Design review of the part built by this model. Coordinates are the model's own, in mm. Face numbers are marked on the shaded views. A direction names the side the tool comes from. Coordinates: 2 decimals unless noted, no trailing zeros. Write each loop counter-clockwise with the first axis right and the second up, starting at its lowest first coordinate (ties: lowest second). Pieces come first, ordered by that corner, then holes. Notation, with made-up numbers: (38, -22.5) - (81, -22.5) arc R9 cw to (81, -15.5) - close; hole circle Ø2 at (59, -27). An arc over 180 degrees is marked (long way). Use a Markdown table: item, result.
from build123d import *

# Parameters (mm, degrees)
SKETCH_1_W          = 36
SKETCH_1_H          = 32
SKETCH_1_R          = 1.6
EXTRUDE_1_DEPTH     = 4
EXTRUDE_2_DEPTH     = 32
SKETCH_8_R          = 1.6
CUT_EXTRUDE_1_DEPTH = 53.619768148
SKETCH1_W           = 4
SKETCH1_H           = 32
BOSS_EXTRUDE1_DEPTH = 3
SKETCH2_W           = 5
SKETCH2_H           = 32
BOSS_EXTRUDE2_DEPTH = 12
CUT_EXTRUDE1_DEPTH  = 5
BOSS_EXTRUDE5_DEPTH = 5
BOSS_EXTRUDE6_START = 3
SKETCH7_W           = 15
SKETCH7_H           = 32
SKETCH7_R           = 1.6
BOSS_EXTRUDE6_DEPTH = 3
CUT_EXTRUDE2_DEPTH  = 0.25
BOSS_EXTRUDE7_START = 2.5
SKETCH9_W           = 15
SKETCH9_H           = 32
SKETCH9_R           = 1.6
BOSS_EXTRUDE7_DEPTH = 2.5
BOSS_EXTRUDE8_DEPTH = 2.5
CUT_EXTRUDE3_DEPTH  = 2.5
FILLET2_R           = 3
FILLET4_R           = 3
FILLET5_R           = 3
FILLET9_R           = 1
FILLET11_R          = 1
CUT_EXTRUDE4_DEPTH  = 3
CUT_EXTRUDE5_DEPTH  = 3
FILLET14_R          = 1


with BuildPart() as part:
    # Эскиз1 → Бобышка-Вытянуть1 (new body)
    with BuildSketch(Plane.XY):
        with Locations((18, 16)):
            Rectangle(SKETCH_1_W, SKETCH_1_H)
        with Locations((8, 26)):
            Circle(SKETCH_1_R, mode=Mode.SUBTRACT)
        with Locations((28, 26)):
            Circle(SKETCH_1_R, mode=Mode.SUBTRACT)
        with Locations((8, 6)):
            Circle(SKETCH_1_R, mode=Mode.SUBTRACT)
        with Locations((28, 6)):
            Circle(SKETCH_1_R, mode=Mode.SUBTRACT)
    extrude(amount=EXTRUDE_1_DEPTH)

    # Эскиз7 → Бобышка-Вытянуть2 (add)
    with BuildSketch(Plane(origin=(0, 32, 0), x_dir=(1, 0, 0), z_dir=(0, 1, 0))):
        Polygon((0, 0), (-1.2, 0), (-1.2, 15), (-5.2, 15), (-5.2, -19), (-1.2, -19), (-1.2, -4), (0, -4), align=None)
    extrude(amount=-EXTRUDE_2_DEPTH)

    # Эскиз8 → Вырез-Вытянуть1 (cut, through all)
    with BuildSketch(Plane(origin=(-1.2, 0, 0), x_dir=(0, 0, -1), z_dir=(1, 0, 0))):
        with Locations(Location((8, 24, 0), (0, 0, 90))):
            Circle(SKETCH_8_R)
        with Locations(Location((8, 8, 0), (0, 0, 90))):
            Circle(SKETCH_8_R)
        with Locations(Location((-12, 8, 0), (0, 0, 90))):
            Circle(SKETCH_8_R)
        with Locations(Location((-12, 24, 0), (0, 0, 90))):
            Circle(SKETCH_8_R)
    extrude(amount=-CUT_EXTRUDE_1_DEPTH, mode=Mode.SUBTRACT)

    # Sketch1 → Boss-Extrude1 (add)
    with BuildSketch(Plane(origin=(36, 0, 0), x_dir=(0, 0, -1), z_dir=(1, 0, 0))):
        with Locations((-2, 16)):
            Rectangle(SKETCH1_W, SKETCH1_H)
    extrude(amount=BOSS_EXTRUDE1_DEPTH)

    # Sketch2 → Boss-Extrude2 (add)
    with BuildSketch(Plane(origin=(0, 0, 0), x_dir=(-1, 0, 0), z_dir=(0, 0, -1))):
        with Locations((-36.5, 16)):
            Rectangle(SKETCH2_W, SKETCH2_H)
    extrude(amount=BOSS_EXTRUDE2_DEPTH)

    # Sketch3 → Cut-Extrude1 (cut)
    with BuildSketch(Plane(origin=(39, 0, 0), x_dir=(0, 0, -1), z_dir=(1, 0, 0))):
        Polygon((7, 32), (12, 32), (12, 23.339745962), align=None)
        Polygon((12, 8.660254038), (7, 0), (12, 0), align=None)
    extrude(amount=-CUT_EXTRUDE1_DEPTH, mode=Mode.SUBTRACT)

    # Sketch6 → Boss-Extrude5 (add)
    with BuildSketch(Plane(origin=(39, 0, 0), x_dir=(0, 0, -1), z_dir=(1, 0, 0))):
        Polygon((-16, 8.660254038), (-11, 0), (-4, 0), (-4, 32), (-11, 32), (-16, 23.339745962), align=None)
    extrude(amount=-BOSS_EXTRUDE5_DEPTH)

    # Sketch7 → Boss-Extrude6 (add)
    # profile 1 of 2: a face of its own
    with BuildSketch(Plane(origin=(-1.2, 0, 0), x_dir=(0, 0, -1), z_dir=(1, 0, 0)).offset(BOSS_EXTRUDE6_START)):
        with Locations((7.5, 16)):
            Rectangle(SKETCH7_W, SKETCH7_H)
        with Locations(Location((8, 24, 0), (0, 0, 90))):
            Circle(SKETCH7_R, mode=Mode.SUBTRACT)
        with Locations(Location((8, 8, 0), (0, 0, 90))):
            Circle(SKETCH7_R, mode=Mode.SUBTRACT)
    # profile 2 of 2: a face of its own
    with BuildSketch(Plane(origin=(-1.2, 0, 0), x_dir=(0, 0, -1), z_dir=(1, 0, 0)).offset(BOSS_EXTRUDE6_START)):
        with Locations((-11.5, 16)):
            Rectangle(SKETCH7_W, SKETCH7_H)
        with Locations(Location((-12, 24, 0), (0, 0, 90))):
            Circle(SKETCH7_R, mode=Mode.SUBTRACT)
        with Locations(Location((-12, 8, 0), (0, 0, 90))):
            Circle(SKETCH7_R, mode=Mode.SUBTRACT)
    extrude(amount=-BOSS_EXTRUDE6_DEPTH)

    # Sketch8 → Cut-Extrude2 (cut)
    with BuildSketch(Plane.ZY.offset(-34)):
        Polygon((-12, 23.339745962), (-12, 8.660254038), (-7, 0), (0, 0), (0, 32), (-7, 32), align=None)
        Polygon((4, 32), (4, 0), (11, 0), (16, 8.660254038), (16, 23.339745962), (11, 32), align=None)
    extrude(amount=-CUT_EXTRUDE2_DEPTH, mode=Mode.SUBTRACT)

    # Sketch9 → Boss-Extrude7 (add)
    with BuildSketch(Plane(origin=(1.8, 0, 0), x_dir=(0, 0, -1), z_dir=(1, 0, 0)).offset(BOSS_EXTRUDE7_START)):
        with Locations((7.5, 16)):
            Rectangle(SKETCH9_W, SKETCH9_H)
        with Locations(Location((8, 24, 0), (0, 0, 90))):
            Circle(SKETCH9_R, mode=Mode.SUBTRACT)
        with Locations(Location((8, 8, 0), (0, 0, 90))):
            Circle(SKETCH9_R, mode=Mode.SUBTRACT)
    extrude(amount=-BOSS_EXTRUDE7_DEPTH)

    # Sketch10 → Boss-Extrude8 (add)
    with BuildSketch(Plane.ZY.offset(-34.25)):
        Polygon((-7, 32), (-12, 23.339745962), (-12, 8.660254038), (-7, 0), (0, 0), (0, 32), align=None)
    extrude(amount=BOSS_EXTRUDE8_DEPTH)

    # Sketch11 → Cut-Extrude3 (cut)
    with BuildSketch(Plane.ZY.offset(-31.75)):
        Polygon((-7, 32), (-12, 23.339745962), (-12, 8.660254038), (-7, 0), align=None)
    extrude(amount=-CUT_EXTRUDE3_DEPTH, mode=Mode.SUBTRACT)

    # Fillet2
    # the kernel refuses this fillet: 3 mm, written as the material it takes off along each edge
    with BuildSketch(Plane(origin=(31.75, -7.395099729, -7), x_dir=(1, 0, 0), z_dir=(0, 1, 0))) as fillet2_piece_1:
        with BuildLine():
            CenterArc((3, -2.958039892), FILLET2_R, 99.594068227, 80.405931773)
            Line((0, -2.958039892), (-0.06, -2.958039892))
            Line((-0.06, -2.958039892), (-0.06, 0))
            Line((-0.06, 0), (0, 0.06))
            ThreePointArc((0, 0.06), (1.25, 0.06), (2.49, 0.059160798))
            Line((2.49, 0.059160798), (2.5, 0))
        make_face()
    extrude(amount=46.790199458, mode=Mode.SUBTRACT)

    # Fillet4
    fillet4_edges = [part.edges().sort_by_distance(p)[0] for p in [
        (36.625, 32, -7),
        (36.625, 0, -7),
        (36.625, 8.660254038, -12),
        (36.625, 23.339745962, -12),
    ]]
    fillet(fillet4_edges, radius=FILLET4_R)

    # Fillet5
    fillet5_edges = [part.edges().sort_by_distance(p)[0] for p in [
        (36.625, 32, 11),
        (36.625, 23.339745962, 16),
        (36.625, 8.660254038, 16),
        (36.625, 0, 11),
    ]]
    fillet(fillet5_edges, radius=FILLET5_R)

    # Fillet9
    fillet9_edges = [part.edges().sort_by_distance(p)[0] for p in [
        (39, 4.732050808, -9.732050808),
        (39, 16, -12),
        (39, 27.267949192, -9.732050808),
        (39, 32, 2),
        (39, 31.598076211, -6.767949192),
        (39, 23.31235552, -11.897777479),
        (39, 8.68764448, -11.897777479),
        (39, 0.401923789, -6.767949192),
        (39, 4.732050808, 13.732050808),
        (39, 0, 2),
        (39, 27.267949192, 13.732050808),
        (39, 16, 16),
        (39, 31.598076211, 10.767949192),
        (39, 23.31235552, 15.897777479),
        (39, 8.68764448, 15.897777479),
        (39, 0.401923789, 10.767949192),
    ]]
    fillet(fillet9_edges, radius=FILLET9_R)

    # Fillet11
    fillet11_edges = [part.edges().sort_by_distance(p)[0] for p in [
        (1.8, 16, 19),
        (-5.2, 16, 19),
        (-1.7, 32, 19),
        (-1.7, 0, 19),
    ]]
    fillet(fillet11_edges, radius=FILLET11_R)

    # Sketch12 → Cut-Extrude4 (cut)
    with BuildSketch(Plane(origin=(4.3, 0, 0), x_dir=(0, 0, -1), z_dir=(1, 0, 0))):
        Polygon((6.354551733, 26.85), (4.709103466, 24), (6.354551733, 21.15), (9.645448267, 21.15), (11.290896534, 24), (9.645448267, 26.85), align=None)
        Polygon((6.354551733, 10.85), (4.709103466, 8), (6.354551733, 5.15), (9.645448267, 5.15), (11.290896534, 8), (9.645448267, 10.85), align=None)
    extrude(amount=-CUT_EXTRUDE4_DEPTH, mode=Mode.SUBTRACT)

    # Sketch13 → Cut-Extrude5 (cut)
    with BuildSketch(Plane(origin=(1.8, 0, 0), x_dir=(0, 0, -1), z_dir=(1, 0, 0))):
        Polygon((-15.290896534, 24), (-13.645448267, 21.15), (-10.354551733, 21.15), (-8.709103466, 24), (-10.354551733, 26.85), (-13.645448267, 26.85), align=None)
        Polygon((-15.290896534, 8), (-13.645448267, 5.15), (-10.354551733, 5.15), (-8.709103466, 8), (-10.354551733, 10.85), (-13.645448267, 10.85), align=None)
    extrude(amount=-CUT_EXTRUDE5_DEPTH, mode=Mode.SUBTRACT)

    # Fillet14
    # the kernel refuses this fillet: 1 mm, written as the material it takes off along each edge
    with BuildSketch(Plane(origin=(-4.2, 1, 18), x_dir=(-1, 0, 0), z_dir=(0, -1, 0))) as fillet14_piece_1_section:
        Polygon((0, 0), (FILLET14_R, 0), (FILLET14_R, -FILLET14_R), (0, -FILLET14_R), align=None)
    fillet14_piece_1 = extrude(amount=FILLET14_R, mode=Mode.PRIVATE)
    fillet14_piece_1 = fillet14_piece_1 - Plane(origin=(-4.2, 1, 18), x_dir=(0.7071067811865475, 0, -0.7071067811865475), z_dir=(0, -1, 0)) * Sphere(FILLET14_R, mode=Mode.PRIVATE)
    add(fillet14_piece_1, mode=Mode.SUBTRACT)
    with BuildSketch(Plane(origin=(-4.2, 31, 18), x_dir=(0, 1, 0), z_dir=(-1, 0, 0))) as fillet14_piece_2_section:
        Polygon((0, 0), (FILLET14_R, 0), (FILLET14_R, -FILLET14_R), (0, -FILLET14_R), align=None)
    fillet14_piece_2 = extrude(amount=FILLET14_R, mode=Mode.PRIVATE)
    fillet14_piece_2 = fillet14_piece_2 - Plane(origin=(-4.2, 31, 18), x_dir=(0, -0.7071067811865475, -0.7071067811865475), z_dir=(-1, 0, 0)) * Sphere(FILLET14_R, mode=Mode.PRIVATE)
    add(fillet14_piece_2, mode=Mode.SUBTRACT)
    with BuildSketch(Plane(origin=(4.3, 32, -17.5), x_dir=(0, -1, 0), z_dir=(0, 0, 1))) as fillet14_piece_3:
        with BuildLine():
            CenterArc((FILLET14_R, -FILLET14_R), FILLET14_R, 90, 90)
            Line((0, -FILLET14_R), (0, 0))
            Line((0, 0), (FILLET14_R, 0))
        make_face()
    extrude(amount=17.5, mode=Mode.SUBTRACT)
    with BuildSketch(Plane(origin=(4.3, 0, 0), x_dir=(-1, 0, 0), z_dir=(0, 0, -1))) as fillet14_piece_4:
        with BuildLine():
            CenterArc((FILLET14_R, FILLET14_R), FILLET14_R, 180, 90)
            Line((0, FILLET14_R), (0, 0))
            Line((0, 0), (FILLET14_R, 0))
        make_face()
    extrude(amount=17.5, mode=Mode.SUBTRACT)
    with BuildSketch(Plane(origin=(4.3, -2.5, -15), x_dir=(-1, 0, 0), z_dir=(0, 1, 0))) as fillet14_piece_5:
        with BuildLine():
            CenterArc((FILLET14_R, FILLET14_R), FILLET14_R, 180, 90)
            Line((0, FILLET14_R), (0, 0))
            Line((0, 0), (FILLET14_R, 0))
        make_face()
    extrude(amount=37, mode=Mode.SUBTRACT)
    with BuildSketch(Plane(origin=(-5.2, 34.5, -15), x_dir=(0, 0, 1), z_dir=(0, -1, 0))) as fillet14_piece_6:
        with BuildLine():
            CenterArc((FILLET14_R, -FILLET14_R), FILLET14_R, 90, 90)
            Line((0, -FILLET14_R), (0, 0))
            Line((0, 0), (FILLET14_R, 0))
        make_face()
    extrude(amount=37, mode=Mode.SUBTRACT)
    with BuildSketch(Plane(origin=(-5.2, 32, -17.5), x_dir=(0, -1, 0), z_dir=(0, 0, 1)), Plane(origin=(-5.2, 0, -17.5), x_dir=(1, 0, 0), z_dir=(0, 0, 1))) as fillet14_piece_7:
        with BuildLine():
            CenterArc((FILLET14_R, FILLET14_R), FILLET14_R, 180, 90)
            Line((0, FILLET14_R), (0, 0))
            Line((0, 0), (FILLET14_R, 0))
        make_face()
    extrude(amount=35.5, mode=Mode.SUBTRACT)


solid = part.part
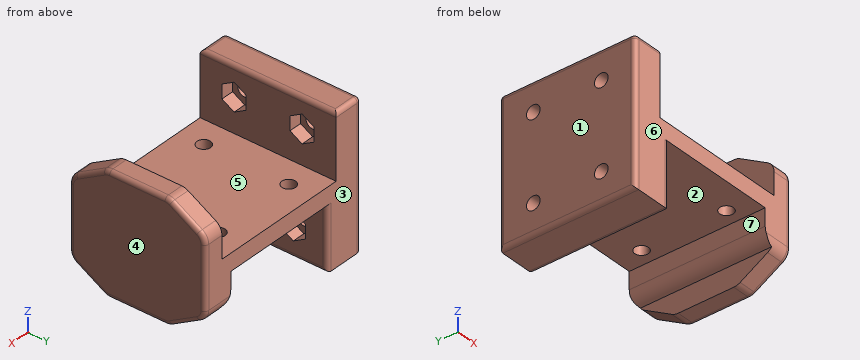
(1) Machinability: for the marked faces 5, 6 and 7, which of the approach directions +Z, -Z, +X, -X, +Y, -Y give a long, thin tool a straight path to every point of the face, cutting with its end or side? Answer none if there is none.
Determined:
| item | result |
|---|---|
| face 5 | +Z, +Y, -Y |
| face 6 | +Z, -Z, +X, -X, -Y |
| face 7 | -Z, +Y, -Y |
(2) For L1, parallel to Z at x = 0.25, y = 24; L2, parallel to Z at x = -3.3, y = 24; L3, parallel to X at y = 26.5, z = -3, list the stretches that pass through material, from the lowest coordinate up. Write a range as from..to.
Determined:
| item | result |
|---|---|
| L1 | -15..-9.6, -6.4..8.71, 15.29..19 |
| L2 | -15..-9.6, -6.4..10.4, 13.6..19 |
| L3 | -5.2..4.3, 31.75..39 |
(3) For pin 1 (5 mm diameter, centred on y = 24, z = -8, fed in from -X); pin 2 (6 mm diameter, centred on x = 9.5, y = 16.5, fed in from -Z); pin 3 (1.5 mm diameter, centred on x = 34, y = 25.5, fed in from -Z); pin 4 (1.1 mm diameter, centred on x = 36, y = 19, fed in from +Z), all flat-tipped, find the tip position at first contact; note any pin that passes through.
Determined:
| item | result |
|---|---|
| pin 1 | x = -5.2 |
| pin 2 | z = 0 |
| pin 3 | z = -11.16 |
| pin 4 | z = 16 |
(4) Draft analysis for pull direction X (two halves, no side actions). For the marked faces 1, 2, 3 and 4, state which applies: +X half, -X half, draft (parallel to the pull), parting line (faces both ways), or undercut.
Determined:
| item | result |
|---|---|
| face 1 | -X half |
| face 2 | undercut |
| face 3 | draft |
| face 4 | +X half |
(5) Take a section at B-B on x = 8. Write out the cut boundary in (y, z), and give its area (3 significant figures).
Determined:
| item | result |
|---|---|
| outline | (0, 0) - (4.4, 0) - (4.4, 4) - (0, 4) - close; (7.6, 0) - (24.4, 0) - (24.4, 4) - (7.6, 4) - close; (27.6, 0) - (32, 0) - (32, 4) - (27.6, 4) - close |
| area | 102 mm2 |
(6) Take a section at C-C on x = 18.5. Write out the cut boundary in (y, z), and give its area (3 significant figures).
Determined:
| item | result |
|---|---|
| outline | (0, 0) - (32, 0) - (32, 4) - (0, 4) - close |
| area | 128 mm2 |
(7) Take a section at A-A on z = 7. Write out the cut boundary in (x, y).
Determined:
| item | result |
|---|---|
| outline | (-5.2, 1) arc R1 ccw to (-4.2, 0) - (1.8, 0) - (1.8, 32) - (-4.2, 32) arc R1 ccw to (-5.2, 31) - close; (34.25, 0) - (38, 0) arc R1 ccw to (39, 1) - (39, 31) arc R1 ccw to (38, 32) - (34.25, 32) - close |
